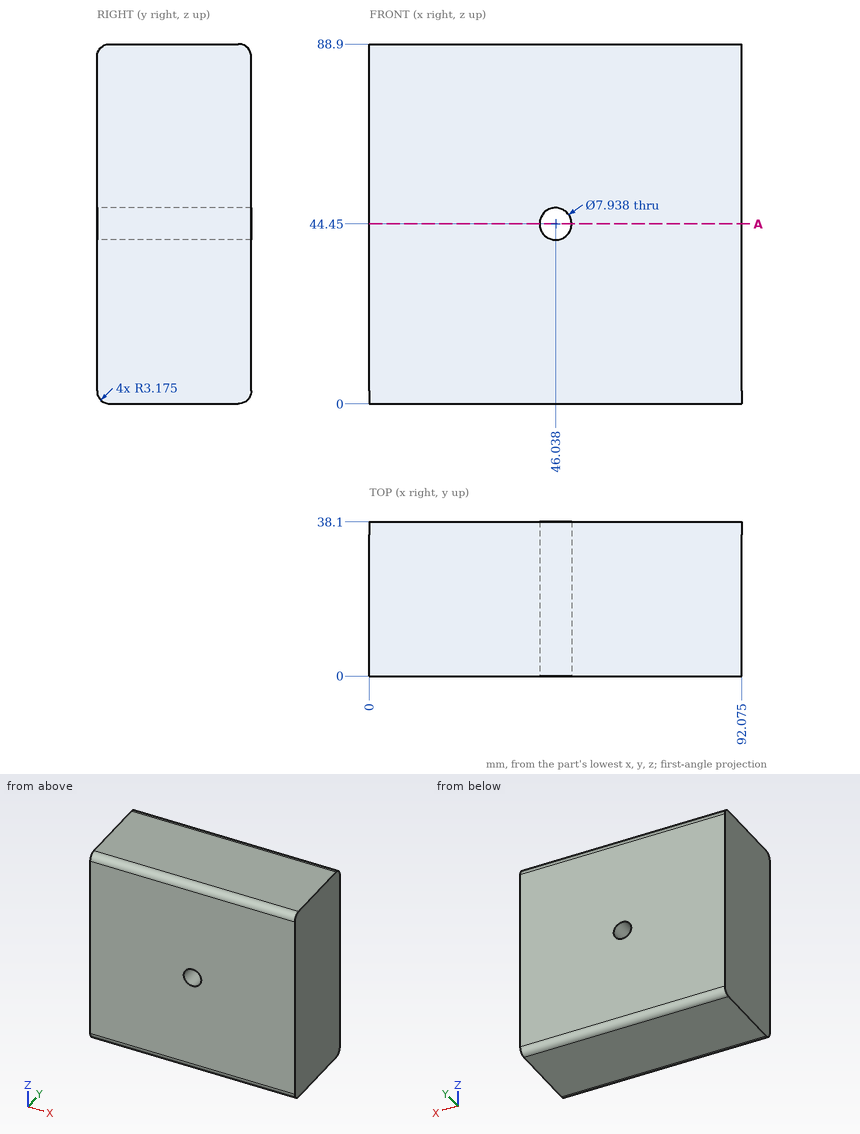
Answer from the drawing. Dimensions are ordinates in mm from the lowest x, y and z of the part. Coordinates: 2 decimals unless noted, no trailing zeros. Order: outer loops, then holes, each group sorted by start corner. A loop starts at its lowest first (then second) coordinate and runs counter-clockwise, first axis right, second up. Notation, with made-up numbers: (58, -32.75) - (65, -32.75) arc R33 ccw to (65, -2.75) - close; hole circle Ø5 at (57, 18). An arc over 180 degrees is marked (long way). Put each result on its own line as item: value. Start each with the question number.
1) Flat-ended cylindrical pins translate along their axes: pin 1 (12 mm diameter, centred on y = 6.5, z = 31, fed in from -X); pin 2 (6.5 mm diameter, centred on x = 46.04, z = 44.45, fed in from +Y) (3 decimals). Find the tip coordinate at first contact, or state that the pin passes through.
2) Find section A-A (z = 44.45). Give the vertices of the cut face in (x, y) (1 decimal).
3) Find the intervals of material crossed by line 1 (X direction, y = 13, z = 44) (1 decimal); line 2 (Z direction, x = 46, y = 23.5); line 3 (Z direction, x = 65, y = 36), in increasing order. Write a range as from..to.
Results list:
1. pin 1: stops at x = 0
1. pin 2: passes through
2. outline: (0, 0) - (42.1, 0) - (42.1, 38.1) - (0, 38.1) - close; (50, 0) - (92.1, 0) - (92.1, 38.1) - (50, 38.1) - close
3. line 1: x = 0..42.1, 50..92.1
3. line 2: z = 0..40.48, 48.42..88.9
3. line 3: z = 0.19..88.71
